Read the model definition and answer for the solid it produces. Units are mm, in the model's axes. A direction names the side the tool comes from. Coordinates: 2 decimals unless noted, no trailing zeros. Order: outer loops, then holes, each group sorted by start corner. A loop starts at its lowest first (then second) coordinate and runs counter-clockwise, first axis right, second up. Notation, with made-up numbers: (-24.5, -39.75) -> (18.5, -39.75) arc R18 cw to (18.5, -27.75) -> close; hole circle Ø4 at (35, 49.5). An arc over 180 degrees is marked (long way). Answer as a JSON object with one key per item and string values. Group by question number.
1) A tool of negligible diameter and unlimited length cuts with its end or side. For faces 4 (the flat face through (-17.05, -68, 2)), 5 (the flat face through (-2, -77.357, 2)), from which of +Z, -Z, +X, -X, +Y, -Y can it reach the whole face along a straight path? Write none if from no direction.
2) Section B-B on y = 10 is taken. Determine the outline of the cut face in (x, z).
3) Section A-A on x = 0 is taken. Determine the outline of the cut face in (y, z).
4) Section D-D on y = 66.5 is taken. Determine the outline of the cut face in (x, z).
5) Consider L1, parallel to Y at x = -26.5, z = 1.4; L2, parallel to X at y = -33.5, z = 0.5; L3, parallel to Y at x = 0, z = 2.6. Determine where each line is inside the solid, lowest interval first.
6) Section C-C on z = 1.3 is taken. Count the separate pieces of the cut face and the enclosed holes in it, and give its area (3 significant figures).
7) Determine the mould class of faces 1 (the flat face through (13.95, -68, 2)), 2 (the flat face through (-36.45, -1, 2)), 3 (the flat face through (-2, 77.357, 2)) for opening direction X: released by +X, released by -X, zero draft, split by the parting line, or undercut.
from build123d import *

# Parameters (mm, degrees)
SKETCH1_W           = 70
SKETCH1_H           = 154.713144252
SKETCH1_R           = 2.4
SKETCH1_R_2         = 2.75
SKETCH1_R_3         = 14
BOSS_EXTRUDE1_DEPTH = 5


with BuildPart() as part:
    # Sketch1 → Boss-Extrude1 (new body)
    with BuildSketch(Plane.XY):
        with Locations((-1.450472168, 0)):
            Rectangle(SKETCH1_W, SKETCH1_H)
        with Locations((-18.5, 57.356572126)):
            Circle(SKETCH1_R, mode=Mode.SUBTRACT)
        with Locations((18.5, 57.356572126)):
            Circle(SKETCH1_R, mode=Mode.SUBTRACT)
        with Locations((-26.450472168, 10)):
            Circle(SKETCH1_R_2, mode=Mode.SUBTRACT)
        with Locations((26.450472168, 10)):
            Circle(SKETCH1_R_2, mode=Mode.SUBTRACT)
        with Locations((26.450472168, -10)):
            Circle(SKETCH1_R_2, mode=Mode.SUBTRACT)
        with Locations((-26.450472168, -10)):
            Circle(SKETCH1_R_2, mode=Mode.SUBTRACT)
        with Locations((0, 57.356572126)):
            Circle(SKETCH1_R_3, mode=Mode.SUBTRACT)
        with BuildLine():
            Line((-13.95, -33.643427874), (-13.95, -40.643427874))
            ThreePointArc((-13.95, -40.643427874), (-15.5, -42.193427874), (-17.05, -40.643427874))
            Line((-17.05, -40.643427874), (-17.05, -33.643427874))
            ThreePointArc((-17.05, -33.643427874), (-15.5, -32.093427874), (-13.95, -33.643427874))
        make_face(mode=Mode.SUBTRACT)
        with BuildLine():
            Line((17.05, -33.643427874), (17.05, -40.643427874))
            ThreePointArc((17.05, -40.643427874), (15.5, -42.193427874), (13.95, -40.643427874))
            Line((13.95, -40.643427874), (13.95, -33.643427874))
            ThreePointArc((13.95, -33.643427874), (15.5, -32.093427874), (17.05, -33.643427874))
        make_face(mode=Mode.SUBTRACT)
        with BuildLine():
            Line((17.05, -64.643427874), (17.05, -71.643427874))
            ThreePointArc((17.05, -71.643427874), (15.5, -73.193427874), (13.95, -71.643427874))
            Line((13.95, -71.643427874), (13.95, -64.643427874))
            ThreePointArc((13.95, -64.643427874), (15.5, -63.093427874), (17.05, -64.643427874))
        make_face(mode=Mode.SUBTRACT)
        with BuildLine():
            Line((-13.95, -64.643427874), (-13.95, -71.643427874))
            ThreePointArc((-13.95, -71.643427874), (-15.5, -73.193427874), (-17.05, -71.643427874))
            Line((-17.05, -71.643427874), (-17.05, -64.643427874))
            ThreePointArc((-17.05, -64.643427874), (-15.5, -63.093427874), (-13.95, -64.643427874))
        make_face(mode=Mode.SUBTRACT)
        with BuildLine():
            Line((-12, -56.143427874), (-12, -49.143427874))
            ThreePointArc((-12, -49.143427874), (0, -37.143427874), (12, -49.143427874))
            Line((12, -49.143427874), (12, -56.143427874))
            ThreePointArc((12, -56.143427874), (0, -68.143427874), (-12, -56.143427874))
        make_face(mode=Mode.SUBTRACT)
    extrude(amount=BOSS_EXTRUDE1_DEPTH)


solid = part.part
Worked answers:
{
 "1": {"face 4": "+Z, -Z", "face 5": "+Z, -Z, +X, -X, -Y"},
 "2": {"outline": "(-36.45, 0) -> (-29.2, 0) -> (-29.2, 5) -> (-36.45, 5) -> close; (-23.7, 0) -> (23.7, 0) -> (23.7, 5) -> (-23.7, 5) -> close; (29.2, 0) -> (33.55, 0) -> (33.55, 5) -> (29.2, 5) -> close"},
 "3": {"outline": "(-77.36, 0) -> (-68.14, 0) -> (-68.14, 5) -> (-77.36, 5) -> close; (-37.14, 0) -> (43.36, 0) -> (43.36, 5) -> (-37.14, 5) -> close; (71.36, 0) -> (77.36, 0) -> (77.36, 5) -> (71.36, 5) -> close"},
 "4": {"outline": "(-36.45, 0) -> (-10.6, 0) -> (-10.6, 5) -> (-36.45, 5) -> close; (10.6, 0) -> (33.55, 0) -> (33.55, 5) -> (10.6, 5) -> close"},
 "5": {"L1": "y = -77.36 to -12.75, -7.25 to 7.25, 12.75 to 77.36", "L2": "x = -36.45 to -17.04, -13.96 to 13.96, 17.04 to 33.55", "L3": "y = -77.36 to -68.14, -37.14 to 43.36, 71.36 to 77.36"},
 "6": {"separate pieces": "1", "enclosed holes": "12", "area": "9,350 mm²"},
 "7": {"face 1": "undercut", "face 2": "released by -X", "face 3": "zero draft"}
}
